from build123d import *

# Parameters (mm, degrees)
SKETCH1_W           = 254
SKETCH1_H           = 25.4
BOSS_EXTRUDE1_DEPTH = 3.175
BOSS_EXTRUDE2_DEPTH = 3.175
SKETCH3_R           = 2.54
CUT_EXTRUDE2_DEPTH  = 4.175


with BuildPart() as part:
    # Sketch1 → Boss-Extrude1 (new body)
    with BuildSketch(Plane(origin=(0, 0, 0), x_dir=(1, 0, 0), z_dir=(0, 1, 0))):
        Rectangle(SKETCH1_W, SKETCH1_H)
    extrude(amount=BOSS_EXTRUDE1_DEPTH)

    # Sketch2 → Boss-Extrude2 (add)
    with BuildSketch(Plane(origin=(0, 3.175, 0), x_dir=(1, 0, 0), z_dir=(0, 1, 0))):
        Polygon((-127, -12.7), (-114.24505896, -42.072282192), (-102.377802862, -19.463351482), (-92.559853535, -42.072282192), (-80.692597436, -19.463351482), (-67.726112797, -42.072282192), (-47.545099388, -19.463351482), (-34.578614749, -42.072282192), (-14.024094064, -24.969728455), (-2.091376305, -39.310937246), (-2.091376305, -24.969728455), (11.649477697, -41.484026388), (20.317707317, -24.969728455), (34.058561319, -41.484026388), (53.714490264, -19.463351482), (63.583568446, -36.671508588), (74.028723274, -24.969728455), (87.13830954, -36.671508588), (101.210719192, -20.906089464), (108.056867206, -36.671508588), (115.76466778, -28.036405605), (119.514469334, -36.671508588), (127, -12.7), align=None)
    extrude(amount=-BOSS_EXTRUDE2_DEPTH)

    # Sketch3 → Cut-Extrude2 (cut, through all)
    with BuildSketch(Plane(origin=(0, 3.175, 0), x_dir=(1, 0, 0), z_dir=(0, 1, 0))):
        with Locations((-114.3, 0)):
            Circle(SKETCH3_R)
        with Locations((114.3, 0)):
            Circle(SKETCH3_R)
    extrude(amount=-CUT_EXTRUDE2_DEPTH, mode=Mode.SUBTRACT)


solid = part.part
Design review of the part built by this model. Coordinates are the model's own, in mm. A direction names the side the tool comes from. Coordinates: 2 decimals unless noted, no trailing zeros. Loops run counter-clockwise (first coordinate to the right, second up) from the corner with the lowest first, then second, coordinate; pieces in that order, holes last. Notation, with made-up numbers: (-10, -25.5) -> (12, -25.5) arc R23 cw to (12, -7.5) -> close; hole circle Ø3 at (-21.5, -18.75). An arc over 180 degrees is marked (long way). Use a Markdown table: item, result. Add a question column.
Item 1: We need section B-B, the plane z = 0. Write out the cut boundary in (x, y) (3 decimals), and give its area (3 significant figures).
Item 2: The part is to be moulded in two halves that separate along Z. For faces 1 (the flat face through (-2, 3.175, 8)), 2 (the cylindrical face through (111.762, 1.61, -0.112)), 3 (the flat face through (-24.445, 1.61, 33.641)), say which applies: +Z half, -Z half, draft (parallel to the pull), parting line (faces both ways), or undercut.
Item 3: We need section C-C, the plane x = -74. Write out the cut boundary in (y, z) (3 decimals).
Item 4: Clearance check with a flat-ended pin moving along its axis: P1, Ø4, axis at x = 114.3, z = 0, coming from the -Y side. State where the tip first meets the part, or that it passes through.
Item 5: We need section A-A, the plane y = 0.6. Write out the cut boundary in (x, z).
Item 6: We need section D-D, the plane z = 30.5. Count the separate pieces of the cut face and the enclosed holes in it, and give its area (3 significant figures).
Item 7: Machinability: for faces 4 (the flat face through (-2, 0, 8)), 5 (the flat face through (43.749, 1.61, 30.628)), which of the approach directions +Z, -Z, +X, -X, +Y, -Y give a long, thin tool a straight path to every point of the face, cutting with its end or side? Answer none if there is none.
Item 8: Wall thickness on L1, parallel to X at y = 0.7, z = 0; L2, parallel to Z at x = -114.3, y = 1.5; L3, parallel to Z at x = 114.3, y = 0.8: over which ranges is each line inside the solid? List them lowest first. Write a range as from..to.
Numbers:
| question | item | result |
|---|---|---|
| 1 | outline | (-127, 0) -> (-116.84, 0) -> (-116.84, 3.175) -> (-127, 3.175) -> close; (-111.76, 0) -> (111.76, 0) -> (111.76, 3.175) -> (-111.76, 3.175) -> close; (116.84, 0) -> (127, 0) -> (127, 3.175) -> (116.84, 3.175) -> close |
| 1 | area | 774 mm^2 |
| 2 | face 1 | draft |
| 2 | face 2 | undercut |
| 2 | face 3 | +Z half |
| 3 | outline | (0, -12.7) -> (3.175, -12.7) -> (3.175, 31.133) -> (0, 31.133) -> close |
| 4 | P1 | passes through |
| 5 | outline | (-127, -12.7) -> (127, -12.7) -> (127, 12.7) -> (119.51, 36.67) -> (115.76, 28.04) -> (108.06, 36.67) -> (101.21, 20.91) -> (87.14, 36.67) -> (74.03, 24.97) -> (63.58, 36.67) -> (53.71, 19.46) -> (34.06, 41.48) -> (20.32, 24.97) -> (11.65, 41.48) -> (-2.09, 24.97) -> (-2.09, 39.31) -> (-14.02, 24.97) -> (-34.58, 42.07) -> (-47.55, 19.46) -> (-67.73, 42.07) -> (-80.69, 19.46) -> (-92.56, 42.07) -> (-102.38, 19.46) -> (-114.25, 42.07) -> (-127, 12.7) -> close; hole circle Ø5.08 at (-114.3, 0); hole circle Ø5.08 at (114.3, 0) |
| 6 | separate pieces | 11 |
| 6 | enclosed holes | 0 |
| 6 | area | 429 mm^2 |
| 7 | face 4 | +Z, -Z, +X, -X, -Y |
| 7 | face 5 | +Z, +Y, -Y |
| 8 | L1 | x = -127..-116.84, -111.76..111.76, 116.84..127 |
| 8 | L2 | z = -12.7..-2.54, 2.54..41.95 |
| 8 | L3 | z = -12.7..-2.54, 2.54..29.68 |
